from build123d import *

# Parameters (mm, degrees)
SKETCH_1_W          = 110
SKETCH_1_H          = 52
EXTRUDE_1_DEPTH     = 4
SKETCH_2_R          = 2.025
CUT_EXTRUDE_1_DEPTH = 4
SKETCH_3_W          = 39.999993186
SKETCH_3_H          = 39
CUT_EXTRUDE_2_DEPTH = 4
FILLET_1_R          = 10


with BuildPart() as part:
    # 草图1 → 凸台-拉伸1 (new body)
    with BuildSketch(Plane.XY):
        Rectangle(SKETCH_1_W, SKETCH_1_H)
    extrude(amount=EXTRUDE_1_DEPTH)

    # 草图2 → 切除-拉伸1 (cut)
    with BuildSketch(Plane(origin=(0, 0, 0), x_dir=(-1, 0, 0), z_dir=(0, 0, -1))):
        with Locations((-47.5, 21)):
            Circle(SKETCH_2_R)
        with Locations((-47.5, 4)):
            Circle(SKETCH_2_R)
        with Locations((-47.5, -21)):
            Circle(SKETCH_2_R)
        with Locations(Location((47.5, -21, 0), (0, 0, 180))):
            Circle(SKETCH_2_R)
        with Locations(Location((47.5, 4, 0), (0, 0, 180))):
            Circle(SKETCH_2_R)
        with Locations(Location((47.5, 21, 0), (0, 0, 180))):
            Circle(SKETCH_2_R)
    extrude(amount=-CUT_EXTRUDE_1_DEPTH, mode=Mode.SUBTRACT)

    # 草图3 → 切除-拉伸2 (cut)
    with BuildSketch(Plane(origin=(0, 0, 0), x_dir=(-1, 0, 0), z_dir=(0, 0, -1))):
        with Locations((3.249996593, 21.45)):
            Rectangle(SKETCH_3_W, SKETCH_3_H)
    extrude(amount=-CUT_EXTRUDE_2_DEPTH, mode=Mode.SUBTRACT)

    # 圆角1
    fillet_1_edges = [part.edges().sort_by_distance(p)[0] for p in [
        (16.75, 1.95, 2),
        (-23.249993186, 1.95, 2),
    ]]
    fillet(fillet_1_edges, radius=FILLET_1_R)


solid = part.part
Build history of the part. All positions in model axes, mm. A direction names the side the tool comes from. Coordinates: 2 decimals unless noted, no trailing zeros. Order: outer loops, then holes, each group sorted by start corner. A loop starts at its lowest first (then second) coordinate and runs counter-clockwise, first axis right, second up. Notation, with made-up numbers: M 25,9.5 L 43,9.5 A21 ccw 43,13.5 Z; hole C 40.25,-20.75 d2. An arc over 180 degrees is marked long. One line per question, with ' | ' between items. Start each with the question number.
Q1. Saw through at C-C (x = 47.5). List the corners of the cut face in (y, z) (3 decimals), then the cut area to 3 significant figures.
Q2. 3-axis set-ups, long thin cutter, end or side, ignore diameter. For faces 4 (the face through (55, 0, 2)), 5 (the face through (13.74, 4.8, 2.03)): which of +Z, -Z, +X, -X, +Y, -Y reach the whole face in a straight line?
Q3. Two-plate mould, pull along X, no slides. Class faces 1 (the face through (16.75, 19, 2)), 2 (the face through (-55, 0, 2)), 3 (the face through (36, 26, 2)): +X half, -X half, draft (parallel to the pull), parting line (faces both ways), or undercut.
Q4. Saw through at A-A (z = 2.4). List the corners of the cut face in (x, y) (3 decimals), then the cut area to 3 significant figures.
Q5. Saw through at B-B (y = 21). List the corners of the cut face in (x, z) (3 decimals).
Q6. Probe L1, parallel to Y at x = 47.5, z = 1.3 (3 decimals); L2, parallel to Y at x = -46, z = 0.35; L3, parallel to X at y = -20.5, z = 3.25. List the from-to ranges inside material, lowest first. Write a range as from..to.
Q7. Saw through at D-D (y = -21). List the corners of the cut face in (x, z) (3 decimals).
Q8. Flat gauge pin, fed straight in: pin 1 Ø3 at (x, y) = (47.5, -21) entering from -Z. Where does the tip first touch, or does it go through?
Check values:
1) outline: M -26,0 L -23.025,0 L -23.025,4 L -26,4 Z; M -18.975,0 L 1.975,0 L 1.975,4 L -18.975,4 Z; M 6.025,0 L 18.975,0 L 18.975,4 L 6.025,4 Z; M 23.025,0 L 26,0 L 26,4 L 23.025,4 Z | area: 159 mm2
2) face 4: +Z, -Z, +X, +Y, -Y | face 5: +Z, -Z, +Y
3) face 1: undercut | face 2: -X half | face 3: draft
4) outline: M -55,-26 L 55,-26 L 55,26 L 16.75,26 L 16.75,11.95 A10 cw 6.75,1.95 L -13.25,1.95 A10 cw -23.25,11.95 L -23.25,26 L -55,26 Z; hole C -47.5,-21 d4.05; hole C -47.5,4 d4.05; hole C -47.5,21 d4.05; hole C 47.5,-21 d4.05; hole C 47.5,4 d4.05; hole C 47.5,21 d4.05 | area: 4,720 mm2
5) outline: M -55,0 L -49.525,0 L -49.525,4 L -55,4 Z; M -45.475,0 L -23.25,0 L -23.25,4 L -45.475,4 Z; M 16.75,0 L 45.475,0 L 45.475,4 L 16.75,4 Z; M 49.525,0 L 55,0 L 55,4 L 49.525,4 Z
6) L1: y = -26..-23.025, -18.975..1.975, 6.025..18.975, 23.025..26 | L2: y = -26..-22.36, -19.64..2.64, 5.36..19.64, 22.36..26 | L3: x = -55..-49.46, -45.54..45.54, 49.46..55
7) outline: M -55,0 L -49.525,0 L -49.525,4 L -55,4 Z; M -45.475,0 L 45.475,0 L 45.475,4 L -45.475,4 Z; M 49.525,0 L 55,0 L 55,4 L 49.525,4 Z
8) pin 1: passes through
